Verification items for the finished model (mm, model axes). A direction names the side the tool comes from. Round coordinates to 2 decimals unless told otherwise and drop trailing zeros. Order: outer loops, then holes, each group sorted by start corner. A loop starts at its lowest first (then second) coordinate and runs counter-clockwise, first axis right, second up. Notation, with made-up numbers: (-18, 77.5) -> (-6, 77.5) arc R19 cw to (-6, 99.5) -> close; hole circle Ø5 at (-23.75, 20). An arc over 180 degrees is marked (long way). Put each result on its own line as item: value.
```python
from build123d import *

# Parameters (mm, degrees)
F0_W     = 38
F0_H     = 48
F1_DEPTH = 25
F3_DEPTH = 50
F4_R     = 3
F5_DEPTH = 12


with BuildPart() as f1:
    # F0 (on Front) → F1 (new body, symmetric)
    with BuildSketch(Plane.XZ):
        with Locations((19, 0)):
            Rectangle(F0_W, F0_H)
    extrude(amount=F1_DEPTH, both=True)

    # F2 (on face) → F3 (cut)
    with BuildSketch(Plane.XZ.offset(25)):
        with BuildLine():
            Line((0, -10), (5.834849, -4))
            ThreePointArc((5.834849, -4), (25, 0), (5.834849, 4))
            Line((5.834849, 4), (0, 10))
            Line((0, 10), (0, -10))
        make_face()
    extrude(amount=-F3_DEPTH, mode=Mode.SUBTRACT)

    # F4 (on face) → F5 (cut)
    with BuildSketch(Plane.YZ.offset(38)):
        with Locations((-17.5, 17.5)):
            Circle(F4_R)
        with Locations((17.5, 17.5)):
            Circle(F4_R)
        with Locations((17.5, -17.5)):
            Circle(F4_R)
        with Locations((-17.5, -17.5)):
            Circle(F4_R)
    extrude(amount=-F5_DEPTH, mode=Mode.SUBTRACT)


solid = f1.part
```
Item 1: Material ranges on line 1 along Z through (x, y) = (32, -17); line 2 along Y through (x, z) = (31, 17); line 3 along Z through (x, y) = (4.5, -21.5), recorded low to high.
Geometry check:
line 1: -24 to -20.46, -14.54 to 14.54, 20.46 to 24
line 2: -25 to -20.46, -14.54 to 14.54, 20.46 to 25
line 3: -24 to -5.37, 5.37 to 24
Item 2: Release check for a two-part mould opening along Y. For faces 1 (the face through (25, 0, 0)), 2 (the face through (27, 25, 0)), 3 (the face through (32.1, 15.1, 15.7)) record: pulls with the +Y half, pulls with the -Y half, needs draft (parallel to the pull), parting line crosses it, or undercut.
Geometry check:
face 1: needs draft
face 2: pulls with the +Y half
face 3: undercut
Item 3: Sectioned sample at D-D, the plane z = -17.5. Record the boundary of the cut face in (x, y), then the cut area to 3 significant figures.
Geometry check:
outline: (0, -25) -> (38, -25) -> (38, -20.5) -> (26, -20.5) -> (26, -14.5) -> (38, -14.5) -> (38, 14.5) -> (26, 14.5) -> (26, 20.5) -> (38, 20.5) -> (38, 25) -> (0, 25) -> close
area: 1,760 mm2
Item 4: Sectioned sample at B-B, the plane y = 17.5. Record the boundary of the cut face in (x, z), then the cut area to 3 significant figures.
Geometry check:
outline: (0, -24) -> (38, -24) -> (38, -20.5) -> (26, -20.5) -> (26, -14.5) -> (38, -14.5) -> (38, 14.5) -> (26, 14.5) -> (26, 20.5) -> (38, 20.5) -> (38, 24) -> (0, 24) -> (0, 10) -> (5.83, 4) arc R10 cw (long way) to (5.83, -4) -> (0, -10) -> close
area: 1,290 mm2
Item 5: Sectioned sample at A-A, the plane x = 29. Record the boundary of the cut face in (y, z), then the cut area to 3 significant figures.
Geometry check:
outline: (-25, -24) -> (25, -24) -> (25, 24) -> (-25, 24) -> close; hole circle Ø6 at (-17.5, -17.5); hole circle Ø6 at (-17.5, 17.5); hole circle Ø6 at (17.5, -17.5); hole circle Ø6 at (17.5, 17.5)
area: 2,290 mm2
Item 6: Depth check by flat-ended pin: pin 1 Ø3 at (y, z) = (17, -17.5) entering from +X; pin 2 Ø18 at (x, z) = (15, 0) entering from +Y; pin 3 Ø1.5 at (y, z) = (-5, -2.5) entering from -X. Enter the tip coordinate at first touch or a pass-through.
Geometry check:
pin 1: x = 26
pin 2: through
pin 3: x = 24.46
Item 7: Sectioned sample at C-C, the plane x = 15. Record the boundary of the cut face in (y, z), then the cut area to 3 significant figures.
Geometry check:
outline: (-25, -24) -> (25, -24) -> (25, -10) -> (-25, -10) -> close; (-25, 10) -> (25, 10) -> (25, 24) -> (-25, 24) -> close
area: 1,400 mm2
Item 8: Tool access check on faces 4 (the face through (26, -18, 18)), 5 (the face through (38, 0, 0)), 6 (the face through (2.88, -0.35, -7.04)). Record the directions out of +Z, -Z, +X, -X, +Y, -Y that give a thin tool (end or side, any length) a straight path to the whole face; none if there is none.
Geometry check:
face 4: +X
face 5: +Z, -Z, +X, +Y, -Y
face 6: -X, +Y, -Y
